Autodesk Inventor part; units mm, degrees
ref_plane "YZ Plane" through (0, 0, 0) normal (1, 0, 0) x (0, 1, 0)
ref_plane "XZ Plane" through (0, 0, 0) normal (0, 1, 0) x (-1, 0, 0)
ref_plane "XY Plane" through (0, 0, 0) normal (0, 0, 1) x (1, 0, 0)
ref_plane "Płaszczyzna konstrukcyjna1" through (0, 0, 0) normal (0, 0, 1) x (1, 0, 0)
sketch "Szkic1" plane through (0, 0, 0) normal (0, 0, 1) x (1, 0, 0)
  line L0 (-7.6801, 0) -> (-5.1801, 0)
  line L1 (-5.1801, 0) -> (18.4779, -65)
  line L2 (18.4779, -65) -> (10.4779, -65)
  arc A0 (10.4779, -65) -> (10.4779, -85) centre (10.4779, -75) ccw
  line L3 (10.4779, -85) -> (80.4779, -85)
  arc A1 (80.4779, -85) -> (80.4779, -65) centre (80.4779, -75) ccw
  line L4 (80.4779, -65) -> (28.4779, -65)
  line L5 (28.4779, -65) -> (4.8199, 0)
  line L6 (4.8199, 0) -> (7.3199, 0)
  line L7 (7.3199, 0) -> (7.3199, 10)
  line L8 (7.3199, 10) -> (-7.6801, 10)
  line L9 (-7.6801, 10) -> (-7.6801, 0)
  point P0 (0, 0)
extrude "Płyta1" add sketch "Szkic1" along normal blind 0.8
equation "\"PromieńGięcia\" = Grubość"
equation "\"SzerokośćGięciaPodcięcia\" = Grubość"
equation "\"GłębokośćGięciaPodcięcia\" = 0.5 * Grubość"
equation "\"RozmiarPodcięciaNarożnika\" = 4 * Grubość"
equation "\"MinimalnaPozostałość\" = 2 * Grubość"
equation "\"PromieńPrzejścia\" = PromieńGięcia"
equation "\"Rozmiar_promienia_Jacobiego\" = Grubość"
equation "\"Wielk_odstępu\" = Grubość"
equation "\"d0\" = PromieńGięcia"
properties part number "club_ABS_metal"
Geometry: final body of the model. Coordinates: model frame, mm. Round coordinates to 2 decimals unless told otherwise and drop trailing zeros. Write each loop counter-clockwise with the first axis right and the second up, starting at its lowest first coordinate (ties: lowest second). Pieces come first, ordered by that corner, then holes.
Item 1: Section query A-A (z = 0.65). Return loops of the section in (x, y).
Item 2: Section query C-C (x = 82). Return loops of the section in (y, z), plus the area to 3 significant figures.
Item 3: Mould query, pull axis Y, two halves, no side actions, for faces 1 (the face through (90.475, -74.78, 0.394)), 2 (the face through (6.48, -32.04, 0.39)), 3 (the face through (33.9, -65.4, 0.8)). Classes: +Y half, -Y half, draft (parallel to the pull), parting line (faces both ways), or undercut.
Item 4: Material intervals for L1, parallel to Y at x = 72, z = 0.35; L2, parallel to X at y = -51.5, z = 0.55; L3, parallel to X at y = -69, z = 0.35, sorted ascending.
Item 5: Section query B-B (y = 3). Return loops of the section in (x, z).
Completed:
1. outline: (-7.68, 0) - (-5.18, 0) - (18.48, -65) - (10.48, -65) arc R10 ccw to (10.48, -85) - (80.48, -85) arc R10 ccw to (80.48, -65) - (28.48, -65) - (4.82, 0) - (7.32, 0) - (7.32, 10) - (-7.68, 10) - close
2. outline: (-84.88, 0) - (-65.12, 0) - (-65.12, 0.8) - (-84.88, 0.8) - close
2. area: 15.8 mm2
3. face 1: parting line
3. face 2: undercut
3. face 3: draft
4. L1: y = -85 to -65
4. L2: x = 13.56 to 23.56
4. L3: x = 2.48 to 88.48
5. outline: (-7.68, 0) - (7.32, 0) - (7.32, 0.8) - (-7.68, 0.8) - close
